Design review of the part built by this model. Coordinates are the model's own, in mm. Face numbers are marked on the shaded views. Coordinates: 2 decimals unless noted, no trailing zeros. Write each loop counter-clockwise with the first axis right and the second up, starting at its lowest first coordinate (ties: lowest second). Pieces come first, ordered by that corner, then holes. Notation, with made-up numbers: M 3.5,68 L 21.5,68 A9 cw 21.5,76 Z; hole C 84,53 d11. An arc over 180 degrees is marked long. Write each question's results on one line, items separated by ' | '. Start each with the question number.
```python
from build123d import *

# Parameters (mm, degrees)
SKETCH1_R           = 38.1
SKETCH1_R_2         = 10.5
BOSS_EXTRUDE1_DEPTH = 20.828
SKETCH6_R           = 17.75000006
CUT_EXTRUDE2_DEPTH  = 1.510000028
SKETCH8_R           = 2.54
CUT_EXTRUDE3_DEPTH  = 42.656
SKETCH9_R           = 14.09889992
CUT_EXTRUDE4_DEPTH  = 0.4


with BuildPart() as part:
    # Sketch1 → Boss-Extrude1 (new body, symmetric)
    with BuildSketch(Plane.XY):
        Circle(SKETCH1_R)
        Circle(SKETCH1_R_2, mode=Mode.SUBTRACT)
    extrude(amount=BOSS_EXTRUDE1_DEPTH, both=True)

    # Sketch6 → Cut-Extrude2 (cut)
    with BuildSketch(Plane(origin=(0, 0, -20.828), x_dir=(-1, 0, 0), z_dir=(0, 0, -1))):
        Circle(SKETCH6_R)
    extrude(amount=-CUT_EXTRUDE2_DEPTH, mode=Mode.SUBTRACT)

    # Sketch8 → Cut-Extrude3 (cut, through all)
    with BuildSketch(Plane.XY.offset(20.828)):
        with Locations((0, 33.3375)):
            Circle(SKETCH8_R)
        with Locations((28.871121899, 16.66875)):
            Circle(SKETCH8_R)
        with Locations((28.871121899, -16.66875)):
            Circle(SKETCH8_R)
        with Locations((0, -33.3375)):
            Circle(SKETCH8_R)
        with Locations((-28.871121899, -16.66875)):
            Circle(SKETCH8_R)
        with Locations((-28.871121899, 16.66875)):
            Circle(SKETCH8_R)
    extrude(amount=-CUT_EXTRUDE3_DEPTH, mode=Mode.SUBTRACT)

    # Sketch9 → Cut-Extrude4 (cut)
    with BuildSketch(Plane(origin=(0, 0, -19.317999972), x_dir=(-1, 0, 0), z_dir=(0, 0, -1))):
        Circle(SKETCH9_R)
    extrude(amount=-CUT_EXTRUDE4_DEPTH, mode=Mode.SUBTRACT)


solid = part.part
```
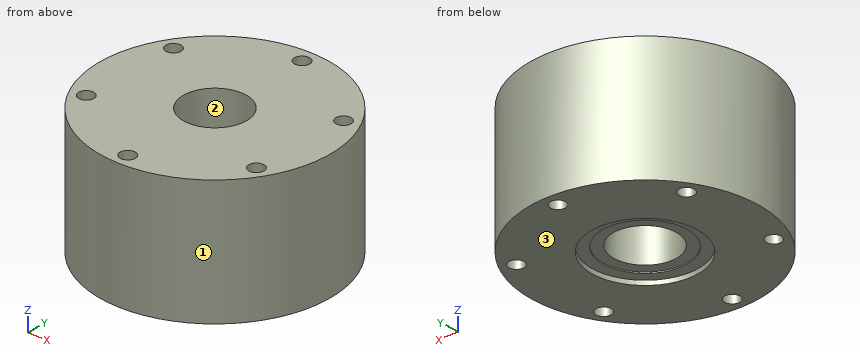
Item 1: We need section C-C on z = -11. State the section outline as (x, y) points.
Item 2: We need section D-D on x = -8.5. State the section outline as (y, z) points, then the cut area to 3 significant figures.
Item 3: Insertion check: pin 1 Ø3 at (x, y) = (28.87, -16.67) entering from +Z; pin 2 Ø2 at (y, z) = (-14.5, -11.5) entering from +X; pin 3 Ø10.5 at (x, y) = (1.5, -6.5) entering from -Z; pin 4 Ø3 at (y, z) = (-12, -3) entering from -X. Each pin has a flat end and moves straight along its axis. Give the tip position at first contact, or say it passes through.
Item 4: Wall thickness on L1, parallel to Y at x = 28.5, z = -1; L2, parallel to X at y = 0.5, z = 2.5; L3, parallel to Y at x = 29, z = 9: over which ranges is each line inside the solid? List them lowest first.
Item 5: We need section A-A on x = 0. State the section outline as (y, z) points.
Item 6: We need section B-B on y = 0. State the section outline as (x, z) points.
Item 7: Draft analysis for pull direction X (two halves, no side actions). For the marked faces 1, 2 and 3, state which applies: released by +X, released by -X, zero draft, split by the parting line, or undercut.
Answer:
1) outline: C 0,0 d76.2; hole C -28.87,-16.67 d5.08; hole C -28.87,16.67 d5.08; hole C 0,0 d21; hole C 0,-33.34 d5.08; hole C 0,33.34 d5.08; hole C 28.87,-16.67 d5.08; hole C 28.87,16.67 d5.08
2) outline: M -37.14,-20.83 L -15.58,-20.83 L -15.58,-19.32 L -11.25,-19.32 L -11.25,-18.92 L -6.16,-18.92 L -6.16,20.83 L -37.14,20.83 Z; M 6.16,-18.92 L 11.25,-18.92 L 11.25,-19.32 L 15.58,-19.32 L 15.58,-20.83 L 37.14,-20.83 L 37.14,20.83 L 6.16,20.83 Z | area: 2,550 mm^2
3) pin 1: passes through | pin 2: stops at x = 35.63 | pin 3: stops at z = -18.92 | pin 4: stops at x = -36.62
4) L1: y = -25.29 to -19.18, -14.16 to 14.16, 19.18 to 25.29 | L2: x = -38.1 to -10.49, 10.49 to 38.1 | L3: y = -24.71 to -19.21, -14.13 to 14.13, 19.21 to 24.71
5) outline: M -38.1,-20.83 L -35.88,-20.83 L -35.88,20.83 L -38.1,20.83 Z; M -30.8,-20.83 L -17.75,-20.83 L -17.75,-19.32 L -14.1,-19.32 L -14.1,-18.92 L -10.5,-18.92 L -10.5,20.83 L -30.8,20.83 Z; M 10.5,-18.92 L 14.1,-18.92 L 14.1,-19.32 L 17.75,-19.32 L 17.75,-20.83 L 30.8,-20.83 L 30.8,20.83 L 10.5,20.83 Z; M 35.88,-20.83 L 38.1,-20.83 L 38.1,20.83 L 35.88,20.83 Z
6) outline: M -38.1,-20.83 L -17.75,-20.83 L -17.75,-19.32 L -14.1,-19.32 L -14.1,-18.92 L -10.5,-18.92 L -10.5,20.83 L -38.1,20.83 Z; M 10.5,-18.92 L 14.1,-18.92 L 14.1,-19.32 L 17.75,-19.32 L 17.75,-20.83 L 38.1,-20.83 L 38.1,20.83 L 10.5,20.83 Z
7) face 1: split by the parting line | face 2: undercut | face 3: zero draft
